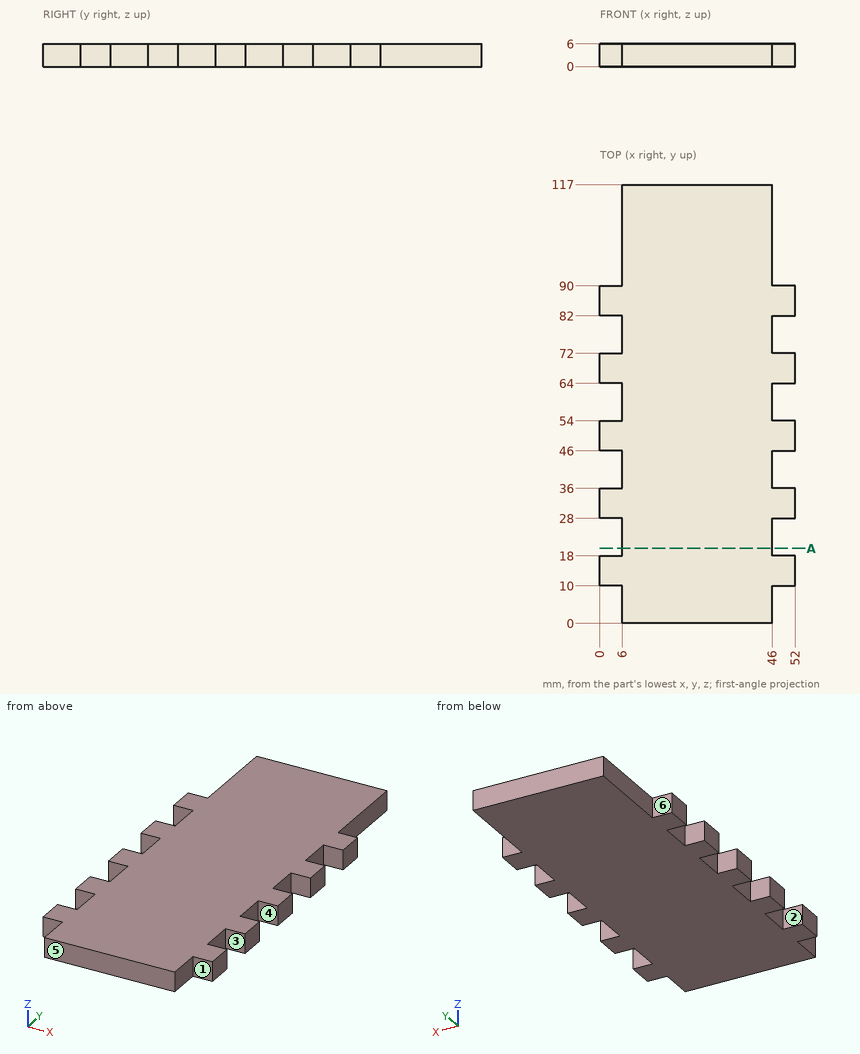
Can you work these out from the drawing? Everything is in mm from the part's minimum corner. A direction names the side the tool comes from. Round coordinates to 2 decimals unless told otherwise and drop trailing zeros. Write each loop counter-clockwise with the first axis right and the second up, starting at its lowest first coordinate (ties: lowest second). Pieces come first, ordered by that corner, then holes. Notation, with made-up numbers: (16.5, 17.5) - (30.5, 17.5) arc R17 ccw to (30.5, 45.5) - close; hole circle Ø10 at (74.5, 10.25). An arc over 180 degrees is marked (long way). Use a Markdown table: item, result.
Q1. For pin 1 (1.8 mm diameter, centred on x = 49, z = 3.5, fed in from -Y); pin 2 (3 mm diameter, centred on x = 50, z = 2.5, fed in from +Y); pin 3 (1.8 mm diameter, centred on y = 21.5, z = 4.5, fed in from -X), each with a flat end and sliding along its axis, tell me the tip position at first contact or that it passes through.
Output values:
| item | result |
|---|---|
| pin 1 | y = 10 |
| pin 2 | y = 90 |
| pin 3 | x = 6 |
Q2. For the marked faces 1, 2 and 3, which set-ups out of +Z, -Z, +X, -X, +Y, -Y let a thin tool reach every point of the face, with its end or its side?
Output values:
| item | result |
|---|---|
| face 1 | +Z, -Z, +X, -Y |
| face 2 | +Z, -Z, -X |
| face 3 | +Z, -Z, +X |
Q3. I want a section at A-A (y = 20). List the corners of the cut face in (x, z) for me.
Output values:
| item | result |
|---|---|
| outline | (6, 0) - (46, 0) - (46, 6) - (6, 6) - close |
Q4. Please list where these lines run through material, in increasing order: L1, parallel to Y at x = 3, z = 0.75; L2, parallel to X at y = 91, z = 4.15.
Output values:
| item | result |
|---|---|
| L1 | 10 to 18, 28 to 36, 46 to 54, 64 to 72, 82 to 90 |
| L2 | 6 to 46 |
Q5. Thinking about a two-plate mould opening in Y: for the marked faces 4, 5 and 6, which applies, released by +Y, released by -Y, zero draft, split by the parting line, or undercut?
Output values:
| item | result |
|---|---|
| face 4 | undercut |
| face 5 | released by -Y |
| face 6 | released by +Y |
